Geometry check sheet. Reference: the model listing, model coordinates, mm. Face numbers are marked on the shaded views. A direction names the side the tool comes from. Round coordinates to 2 decimals unless told otherwise and drop trailing zeros. Order: outer loops, then holes, each group sorted by start corner. A loop starts at its lowest first (then second) coordinate and runs counter-clockwise, first axis right, second up. Notation, with made-up numbers: (-11.75, -31) -> (16.25, -31) arc R8 cw to (16.25, -22) -> close; hole circle Ø9 at (-33.75, 82). An arc over 180 degrees is marked (long way). Answer as a JSON object with one key per item and string values. Group by question number.
from build123d import *

# Parameters (mm, degrees)
F1_DEPTH = 700
F2_W     = 500
F2_H     = 450
F3_DEPTH = 600
F5_DEPTH = 600.001
F6_W     = 620
F6_H     = 100
F7_DEPTH = 900.001


with BuildPart() as f1:
    # F0 (on Front) → F1 (new body)
    with BuildSketch(Plane.XZ):
        Polygon((0, 980), (0, 0), (40, 0), (40, 120), (860, 120), (860, 0), (900, 0), (900, 700), (700, 980), align=None)
    extrude(amount=F1_DEPTH)

    # F2 (on face) → F3 (join)
    with BuildSketch(Plane.YZ.offset(900)):
        with Locations((-350, 375)):
            Rectangle(F2_W, F2_H)
    extrude(amount=F3_DEPTH)

    # F4 (on face) → F5 (cut, through all)
    with BuildSketch(Plane.XZ.offset(600)):
        Polygon((1500, 450), (1500, 600), (1300, 600), align=None)
    extrude(amount=-F5_DEPTH, mode=Mode.SUBTRACT)

    # F6 (on face) → F7 (cut, through all)
    with BuildSketch(Plane.YZ.offset(900)):
        with Locations((-350, 50)):
            Rectangle(F6_W, F6_H)
    extrude(amount=-F7_DEPTH, mode=Mode.SUBTRACT)


solid = f1.part
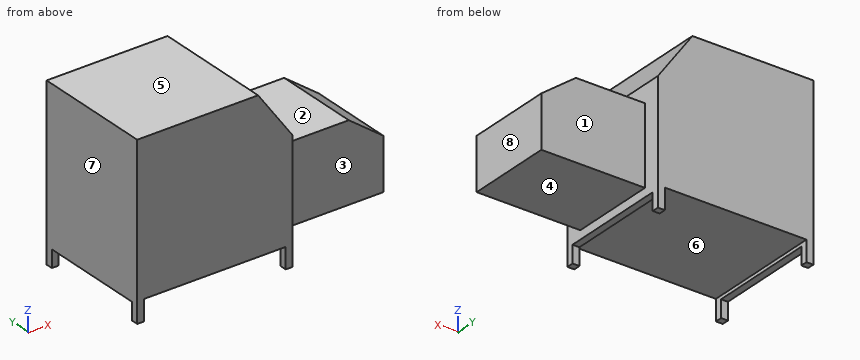
Item 1: Set-up check for the marked faces 1, 2, 3 and 4: record each of +Z, -Z, +X, -X, +Y, -Y from which the full face is reachable in a straight line by a thin tool's end or side.
Item 2: Sectioned sample at D-D, the plane x = 672. Enter the section's corners in (y, z).
Item 3: Depth check by flat-ended pin: pin 1 Ø12 at (x, y) = (13.5, -348.5) entering from -Z; pin 2 Ø2 at (y, z) = (-413.5, 689.5) entering from +X. Enter the tip coordinate at first touch or a pass-through.
Item 4: Sectioned sample at B-B, the plane y = -344. Enter the section's corners in (x, z), then the cut area to 3 significant figures.
Item 5: Mould release check, pull along X, two halves, no side actions. Record for the marked faces 5, 6, 7 and 8: pulls with the +X half, pulls with the -X half, needs draft (parallel to the pull), parting line crosses it, or undercut.
Item 6: Sectioned sample at C-C, the plane z = 299.5. Enter the section's corners in (x, y).
Item 7: Sectioned sample at A-A, the plane z = 82.5. Enter the section's corners in (x, y).
Item 8: Thickness scan on L1, parallel to Y at x = 1115, z = 401.5; L2, parallel to Z at x = 454, y = -557; L3, parallel to Z at x = 1025, y = -506. Record the ranges inside material, lowest first.
Result:
{
 "1": {"face 1": "+Z, -Z, +X, +Y", "face 2": "+Z, +X, +Y, -Y", "face 3": "+Z, -Z, +X, -Y", "face 4": "-Z, +X, +Y, -Y"},
 "2": {"outline": "(-700, 120) -> (0, 120) -> (0, 980) -> (-700, 980) -> close"},
 "3": {"pin 1": "stops at z = 100", "pin 2": "stops at x = 900"},
 "4": {"outline": "(0, 100) -> (40, 100) -> (40, 120) -> (860, 120) -> (860, 100) -> (900, 100) -> (900, 150) -> (1500, 150) -> (1500, 450) -> (1300, 600) -> (900, 600) -> (900, 700) -> (700, 980) -> (0, 980) -> close", "area": "1,000,000 mm2"},
 "5": {"face 5": "needs draft", "face 6": "undercut", "face 7": "pulls with the -X half", "face 8": "pulls with the +X half"},
 "6": {"outline": "(0, -700) -> (900, -700) -> (900, -600) -> (1500, -600) -> (1500, -100) -> (900, -100) -> (900, 0) -> (0, 0) -> close"},
 "7": {"outline": "(0, -700) -> (40, -700) -> (40, -660) -> (0, -660) -> close; (0, -40) -> (40, -40) -> (40, 0) -> (0, 0) -> close; (860, -700) -> (900, -700) -> (900, -660) -> (860, -660) -> close; (860, -40) -> (900, -40) -> (900, 0) -> (860, 0) -> close"},
 "8": {"L1": "y = -600 to -100", "L2": "z = 120 to 980", "L3": "z = 150 to 600"}
}
